Geometry check sheet. Reference: the model listing, model coordinates, mm. A direction names the side the tool comes from. Give positions to 0.01 mm unless a question says otherwise; leave off trailing zeros. Write each loop counter-clockwise with the first axis right and the second up, starting at its lowest first coordinate (ties: lowest second). Pieces come first, ordered by that corner, then holes.
(1) Cross-section at A-A (x = -54). Record the boundary of the cut face in (y, z), and give its area (3 significant figures).
(2) Tool access check on faces 1 (the flat face through (0, -12.5, 20)), 2 (the flat face through (-26.04, -8.82, 8.58)), 3 (the cylindrical face through (-1.804, 0.175, 20.289)). Record the directions out of +Z, -Z, +X, -X, +Y, -Y that give a thin tool (end or side, any length) a straight path to the whole face; none if there is none.
(3) Cross-section at B-B (x = -27.5). Record the boundary of the cut face in (y, z).
(4) Depth check by flat-ended pin: P1, Ø2, axis at y = -12.5, z = 13, coming from the +X side; P2, Ø3, axis at x = -44.5, y = -1.5, coming from the -Z side; P3, Ø7.5, axis at y = 4.5, z = 6.5, coming from the -X side. Enter the tip coordinate at first touch or a pass-through.
(5) Cross-section at D-D (x = -4). Record the boundary of the cut face in (y, z), and give its area (3 significant figures).
(6) Thickness scan on line 1 along Y through (x, z) = (1, 0); line 2 along X through (y, z) = (-15, 13); line 3 along Z through (x, y) = (-9, 0.5). Record the ranges inside material, lowest first.
(7) Cross-section at C-C (y = -18). Record the boundary of the cut face in (x, z).
```python
from build123d import *

# Parameters (mm, degrees)
SKETCH1_R           = 12.5
SKETCH1_R_2         = 7.5
BOSS_EXTRUDE1_DEPTH = 12
SKETCH1_3_R         = 7.5
SKETCH1_3_R_2       = 4
BOSS_EXTRUDE2_DEPTH = 4
SKETCH2_W           = 12
SKETCH2_H           = 25
BOSS_EXTRUDE3_DEPTH = 32
CUT_EXTRUDE1_DEPTH  = 8
CUT_EXTRUDE2_DEPTH  = 13
SKETCH4_W           = 10
SKETCH4_H           = 25
BOSS_EXTRUDE4_DEPTH = 72
FILLET1_R           = 6
FILLET2_R           = 10
FILLET3_R           = 4
SKETCH5_W           = 6
SKETCH5_H           = 30.078064569
BOSS_EXTRUDE5_DEPTH = 35
CUT_EXTRUDE3_REACH  = 43
SKETCH7_W           = 6
SKETCH7_H           = 17.578064569
BOSS_EXTRUDE6_DEPTH = 6
CUT_EXTRUDE4_REACH  = 43
FILLET4_R           = 5


with BuildPart() as part:
    # Sketch1 → Boss-Extrude1 (new body)
    with BuildSketch(Plane(origin=(0, 0, 0), x_dir=(0, 0, -1), z_dir=(1, 0, 0))):
        Circle(SKETCH1_R)
        Circle(SKETCH1_R_2, mode=Mode.SUBTRACT)
    extrude(amount=BOSS_EXTRUDE1_DEPTH)

    # Sketch1<3> → Boss-Extrude2 (add)
    with BuildSketch(Plane(origin=(0, 0, 0), x_dir=(0, 0, -1), z_dir=(1, 0, 0))):
        Circle(SKETCH1_3_R)
        Circle(SKETCH1_3_R_2, mode=Mode.SUBTRACT)
    extrude(amount=BOSS_EXTRUDE2_DEPTH)

    # Sketch2 → Boss-Extrude3 (add)
    with BuildSketch(Plane.XY):
        with Locations((6, 0)):
            Rectangle(SKETCH2_W, SKETCH2_H)
    extrude(amount=BOSS_EXTRUDE3_DEPTH)

    # Sketch3 → Cut-Extrude1 (cut)
    with BuildSketch(Plane(origin=(12, 0, -12), x_dir=(0, 0, 1), z_dir=(-1, 0, 0))):
        with BuildLine():
            ThreePointArc((12, 4), (14.828427125, 2.828427125), (16, 0))
            ThreePointArc((16, 0), (14.828427125, -2.828427125), (12, -4))
            Line((12, -4), (12, -7.5))
            ThreePointArc((12, -7.5), (17.303300859, -5.303300859), (19.5, 0))
            ThreePointArc((19.5, 0), (17.303300859, 5.303300859), (12, 7.5))
            Line((12, 7.5), (12, 4))
        make_face()
        with BuildLine():
            ThreePointArc((12, -4), (8, 0), (12, 4))
            Line((12, 4), (12, 7.5))
            ThreePointArc((12, 7.5), (4.5, 0), (12, -7.5))
            Line((12, -7.5), (12, -4))
        make_face()
    extrude(amount=CUT_EXTRUDE1_DEPTH, mode=Mode.SUBTRACT)

    # Sketch3<6> → Cut-Extrude2 (cut, through all)
    with BuildSketch(Plane(origin=(12, 0, -12), x_dir=(0, 0, 1), z_dir=(-1, 0, 0))):
        with BuildLine():
            ThreePointArc((12, -4), (14.828427125, -2.828427125), (16, 0))
            ThreePointArc((16, 0), (14.828427125, 2.828427125), (12, 4))
            Line((12, 4), (12, -4))
        make_face()
        with BuildLine():
            Line((12, -4), (12, 4))
            ThreePointArc((12, 4), (8, 0), (12, -4))
        make_face()
    extrude(amount=CUT_EXTRUDE2_DEPTH, mode=Mode.SUBTRACT)

    # Sketch4 → Boss-Extrude4 (add)
    with BuildSketch(Plane.ZY):
        with Locations((27, 0)):
            Rectangle(SKETCH4_W, SKETCH4_H)
    extrude(amount=BOSS_EXTRUDE4_DEPTH)

    # Fillet1
    fillet1_edges = [part.edges().sort_by_distance(p)[0] for p in [
        (0, 0, 22),
    ]]
    fillet(fillet1_edges, radius=FILLET1_R)

    # Fillet2
    fillet2_edges = [part.edges().sort_by_distance(p)[0] for p in [
        (12, 0, 32),
    ]]
    fillet(fillet2_edges, radius=FILLET2_R)

    # Fillet3
    fillet3_edges = [part.edges().sort_by_distance(p)[0] for p in [
        (9.071067812, -12.5, 29.071067812),
        (12, 0, -12.5),
        (-36, -12.5, 32),
        (-72, 0, 32),
        (-72, 12.5, 27),
        (-72, -12.5, 27),
        (-36, 12.5, 32),
        (12, 12.5, 11),
        (9.071067812, 12.5, 29.071067812),
        (12, -12.5, 11),
    ]]
    fillet(fillet3_edges, radius=FILLET3_R)

    # Sketch5 → Boss-Extrude5 (add)
    with BuildSketch(Plane(origin=(0, 0, 22), x_dir=(-1, 0, 0), z_dir=(0, 0, -1))):
        with Locations((26, -15.039032285)):
            Rectangle(SKETCH5_W, SKETCH5_H)
    extrude(amount=BOSS_EXTRUDE5_DEPTH)

    # Sketch6 → Cut-Extrude3 (cut, up to next)
    with BuildSketch(Plane.ZY.offset(29), mode=Mode.PRIVATE) as cut_extrude3_sk1:
        Polygon((-4.627390911, -30.078064569), (14.060102478, 0), (-13, 0), (-13, -30.078064569), align=None)
    cut_extrude3_tool1 = extrude(cut_extrude3_sk1.sketch, amount=-CUT_EXTRUDE3_REACH, mode=Mode.PRIVATE) & part.part
    add(cut_extrude3_tool1.solids().sort_by_distance((-29, -12.395131, -3.320494))[0], mode=Mode.SUBTRACT)

    # Sketch7 → Boss-Extrude6 (add)
    with BuildSketch(Plane.XY.offset(22)):
        with Locations((-26, -21.289032285)):
            Rectangle(SKETCH7_W, SKETCH7_H)
    extrude(amount=BOSS_EXTRUDE6_DEPTH)

    # Sketch8 → Cut-Extrude4 (cut, up to next)
    with BuildSketch(Plane.ZY.offset(29), mode=Mode.PRIVATE) as cut_extrude4_sk1:
        Polygon((28, -12.5), (21.643434009, -22.731077991), (-0.062710135, -22.731077991), (-4.627390911, -30.078064569), (28, -30.078064569), align=None)
    cut_extrude4_tool1 = extrude(cut_extrude4_sk1.sketch, amount=-CUT_EXTRUDE4_REACH, mode=Mode.PRIVATE) & part.part
    add(cut_extrude4_tool1.solids().sort_by_distance((-29, -25.583256, 14.464083))[0], mode=Mode.SUBTRACT)

    # Fillet4
    fillet4_edges = [part.edges().sort_by_distance(p)[0] for p in [
        (-26, 0, 14.060102478),
        (-26, -22.731077991, -0.062710135),
        (-26, -22.731077991, 21.643434009),
    ]]
    fillet(fillet4_edges, radius=FILLET4_R)


solid = part.part
```
Reply:
1. outline: (-12.5, 22) - (12.5, 22) - (12.5, 28) arc R4 ccw to (8.5, 32) - (-8.5, 32) arc R4 ccw to (-12.5, 28) - close
1. area: 243 mm2
2. face 1: +Z, -Z, +X, -Y
2. face 2: -Z, -X, +Y
2. face 3: -Z, +Y, -Y
3. outline: (-22.73, 8.93) arc R5 ccw to (-15.09, 4.68) - (-2.36, 12.59) arc R5 ccw to (0, 16.84) - (0, 22) - (12.5, 22) - (12.5, 28) arc R4 ccw to (8.5, 32) - (-8.5, 32) arc R4 ccw to (-12.5, 28) - (-20.37, 23.11) arc R5 ccw to (-22.73, 18.86) - close
4. P1: stops at x = 10.65
4. P2: stops at z = 22
4. P3: stops at x = 0
5. outline: (-12.5, 21.66) - (12.5, 21.66) - (12.5, 28) arc R4 ccw to (8.5, 32) - (-8.5, 32) arc R4 ccw to (-12.5, 28) - close
5. area: 252 mm2
6. line 1: y = -12.5 to -4, 4 to 12.5
6. line 2: x = -29 to -23
6. line 3: z = 22 to 32
7. outline: (-29, 3.94) - (-23, 3.94) - (-23, 24.58) - (-29, 24.58) - close
